Job drawing, mm, ordinate dimensions from the low corner. One solid piece. Give positions to 0.01 mm unless a question says otherwise; leave off trailing zeros. Order: outer loops, then holes, each group sorted by start corner. A loop starts at its lowest first (then second) coordinate and runs counter-clockwise, first axis right, second up.
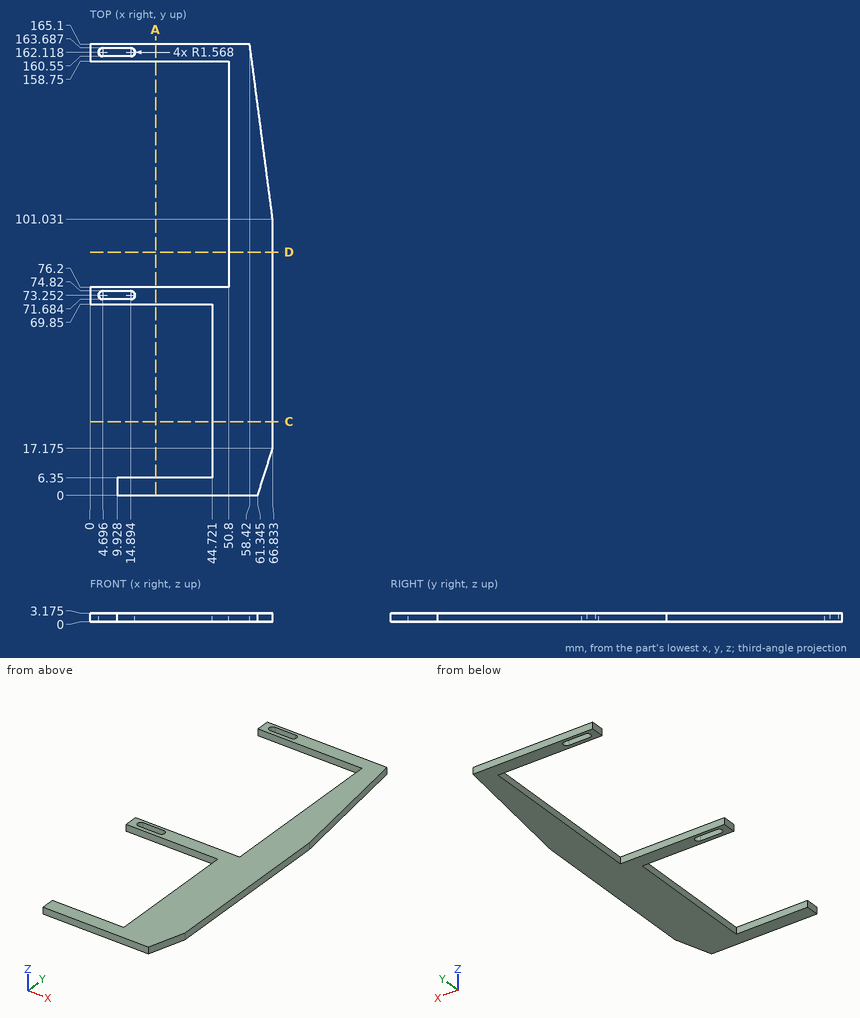
Item 1: Drill centre lines: probe 1 along Y at (x, z) = (6.5, 0.8); probe 2 along Y at (x, z) = (13, 2.65); probe 3 along Y at (x, z) = (42, 0.65). Where is each one in solid material? Low to high.
Item 2: Band-saw the part on A-A on x = 24. Give the number of separate pieces and of enclosed holes in the cut face.
Item 3: Drop flat-ended pins along their axis: P1, Ø1.6, axis at y = 48, z = 2, coming from the -X side; P2, Ø1.6, axis at y = 3, z = 1.5, coming from the -X side. Give the stop position or say it passes through.
Item 4: Band-saw the part on C-C on y = 27. List the corners of the cut face in (x, z) (1 decimal).
Item 5: Band-saw the part on D-D on y = 89. List the corners of the cut face in (x, z) (1 decimal), plus the area to 3 significant figures.
Working result:
1. probe 1: y = 69.85 to 71.68, 74.82 to 76.2, 158.75 to 160.55, 163.69 to 165.1
1. probe 2: y = 0 to 6.35, 69.85 to 71.68, 74.82 to 76.2, 158.75 to 160.55, 163.69 to 165.1
1. probe 3: y = 0 to 6.35, 69.85 to 76.2, 158.75 to 165.1
2. separate pieces: 3
2. enclosed holes: 0
3. P1: stops at x = 44.72
3. P2: stops at x = 9.93
4. outline: (44.7, 0) - (66.8, 0) - (66.8, 3.2) - (44.7, 3.2) - close
5. outline: (50.8, 0) - (66.8, 0) - (66.8, 3.2) - (50.8, 3.2) - close
5. area: 50.9 mm2
